```python
from build123d import *

# Parameters (mm, degrees)
SKETCH_1_W             = 6
SKETCH_1_H             = 43
EXTRUDE_1_DEPTH        = 10
SKETCH_3_R             = 1
EXTRUDE_2_DEPTH        = 3
FILLET_1_R             = 1
SKETCH_4_W             = 0.5
SKETCH_4_H             = 2
SKETCH_4_W_2           = 2
SKETCH_4_H_2           = 0.5
CUT_EXTRUDE_1_DEPTH    = 4
SKETCH_5_OUTSIDE_W     = 17.062
SKETCH_5_OUTSIDE_H     = 54.062
CUT_EXTRUDE_2_DEPTH    = 7
CUT_EXTRUDE_3_DEPTH    = 7
SKETCH_7_W             = 3.5
SKETCH_7_H             = 36
CUT_EXTRUDE_4_DEPTH    = 2
CHAMFER_1_SIZE         = 2
CHAMFER_1_SIZE2        = 0.5
CHAMFER_1_PART_2_SIZE  = 2
CHAMFER_1_PART_2_SIZE2 = 0.5
CHAMFER_2_SIZE         = 2
CHAMFER_2_SIZE2        = 0.5
CHAMFER_2_PART_2_SIZE  = 2
CHAMFER_2_PART_2_SIZE2 = 0.5
CHAMFER_3_SIZE         = 2
CHAMFER_3_SIZE2        = 1
CHAMFER_3_PART_2_SIZE  = 2
CHAMFER_3_PART_2_SIZE2 = 1
CHAMFER_4_SIZE         = 0.5
CHAMFER_4_SIZE2        = 1
CHAMFER_4_PART_2_SIZE  = 0.5
CHAMFER_4_PART_2_SIZE2 = 1


with BuildPart() as part:
    # 草图1 → 凸台-拉伸1 (new body)
    with BuildSketch(Plane(origin=(0, 0, 0), x_dir=(1, 0, 0), z_dir=(0, 1, 0))):
        Rectangle(SKETCH_1_W, SKETCH_1_H)
    extrude(amount=EXTRUDE_1_DEPTH)

    # 草图3 → 凸台-拉伸2 (add)
    with BuildSketch(Plane.XZ):
        with Locations((0, 19.5)):
            Circle(SKETCH_3_R)
        with Locations((0, -19.5)):
            Circle(SKETCH_3_R)
    extrude(amount=EXTRUDE_2_DEPTH)

    # 圆角1
    fillet_1_edges = [part.edges().sort_by_distance(p)[0] for p in [
        (-1, -3, 19.5),
        (-1, -3, -19.5),
    ]]
    fillet(fillet_1_edges, radius=FILLET_1_R)

    # 草图4 → 切除-拉伸1 (cut, through all)
    with BuildSketch(Plane.XZ):
        with Locations((0, 19.5)):
            Rectangle(SKETCH_4_W, SKETCH_4_H)
        with Locations((0, -19.5)):
            Rectangle(SKETCH_4_W_2, SKETCH_4_H_2)
    extrude(amount=CUT_EXTRUDE_1_DEPTH, mode=Mode.SUBTRACT)

    # 草图5 outside → 切除-拉伸2 (cut)
    with BuildSketch(Plane(origin=(0, 10, 0), x_dir=(1, 0, 0), z_dir=(0, 1, 0))):
        Rectangle(SKETCH_5_OUTSIDE_W, SKETCH_5_OUTSIDE_H)
        Polygon((-0.75, -20.25), (0.75, -20.25), (0.75, -18), (1.75, -18), (1.75, 18), (0.75, 18), (0.75, 20.25), (-0.75, 20.25), (-0.75, 18), (-1.75, 18), (-1.75, -18), (-0.75, -18), align=None, mode=Mode.SUBTRACT)
    extrude(amount=-CUT_EXTRUDE_2_DEPTH, mode=Mode.SUBTRACT)

    # 草图6 → 切除-拉伸3 (cut)
    with BuildSketch(Plane(origin=(0, 10, 0), x_dir=(1, 0, 0), z_dir=(0, 1, 0))):
        Polygon((-1.25, 17), (0.25, 17), (0.25, -2.5), (1.45, -2.5), (1.45, -4), (-1.25, -4), align=None)
        Polygon((-1.25, -17), (0.25, -17), (0.25, -7.5), (1.45, -7.5), (1.45, -6), (-1.25, -6), align=None)
    extrude(amount=-CUT_EXTRUDE_3_DEPTH, mode=Mode.SUBTRACT)

    # 草图7 → 切除-拉伸4 (cut)
    with BuildSketch(Plane(origin=(0, 10, 0), x_dir=(1, 0, 0), z_dir=(0, 1, 0))):
        Rectangle(SKETCH_7_W, SKETCH_7_H)
    extrude(amount=-CUT_EXTRUDE_4_DEPTH, mode=Mode.SUBTRACT)

    # 倒角1
    chamfer_1_edges = [part.edges().sort_by_distance(p)[0] for p in [
        (0.75, 10, -19.125),
    ]]
    chamfer_1_side = [part.faces().sort_by_distance(p)[0] for p in [
        (0.75, 6.5, -19.125),
    ]]
    chamfer(chamfer_1_edges, length=CHAMFER_1_SIZE, length2=CHAMFER_1_SIZE2, reference=chamfer_1_side[0])

    # 倒角1 part 2
    chamfer_1_part_2_edges = [part.edges().sort_by_distance(p)[0] for p in [
        (-0.75, 10, -19.125),
    ]]
    chamfer_1_part_2_side = [part.faces().sort_by_distance(p)[0] for p in [
        (-0.75, 6.5, -19.125),
    ]]
    chamfer(chamfer_1_part_2_edges, length=CHAMFER_1_PART_2_SIZE, length2=CHAMFER_1_PART_2_SIZE2, reference=chamfer_1_part_2_side[0])

    # 倒角2
    chamfer_2_edges = [part.edges().sort_by_distance(p)[0] for p in [
        (0.75, 10, 19.125),
    ]]
    chamfer_2_side = [part.faces().sort_by_distance(p)[0] for p in [
        (0.75, 6.5, 19.125),
    ]]
    chamfer(chamfer_2_edges, length=CHAMFER_2_SIZE, length2=CHAMFER_2_SIZE2, reference=chamfer_2_side[0])

    # 倒角2 part 2
    chamfer_2_part_2_edges = [part.edges().sort_by_distance(p)[0] for p in [
        (-0.75, 10, 19.125),
    ]]
    chamfer_2_part_2_side = [part.faces().sort_by_distance(p)[0] for p in [
        (-0.75, 6.5, 19.125),
    ]]
    chamfer(chamfer_2_part_2_edges, length=CHAMFER_2_PART_2_SIZE, length2=CHAMFER_2_PART_2_SIZE2, reference=chamfer_2_part_2_side[0])

    # 倒角3
    chamfer_3_edges = [part.edges().sort_by_distance(p)[0] for p in [
        (0, 10, -20.25),
    ]]
    chamfer_3_side = [part.faces().sort_by_distance(p)[0] for p in [
        (0, 6.201754386, -20.25),
    ]]
    chamfer(chamfer_3_edges, length=CHAMFER_3_SIZE, length2=CHAMFER_3_SIZE2, reference=chamfer_3_side[0])

    # 倒角3 part 2
    chamfer_3_part_2_edges = [part.edges().sort_by_distance(p)[0] for p in [
        (0, 10, 20.25),
    ]]
    chamfer_3_part_2_side = [part.faces().sort_by_distance(p)[0] for p in [
        (0, 6.201754386, 20.25),
    ]]
    chamfer(chamfer_3_part_2_edges, length=CHAMFER_3_PART_2_SIZE, length2=CHAMFER_3_PART_2_SIZE2, reference=chamfer_3_part_2_side[0])

    # 倒角4
    chamfer_4_edges = [part.edges().sort_by_distance(p)[0] for p in [
        (0, 10, -18),
    ]]
    chamfer_4_side = [part.faces().sort_by_distance(p)[0] for p in [
        (0, 10, -18.625),
    ]]
    chamfer(chamfer_4_edges, length=CHAMFER_4_SIZE, length2=CHAMFER_4_SIZE2, reference=chamfer_4_side[0])

    # 倒角4 part 2
    chamfer_4_part_2_edges = [part.edges().sort_by_distance(p)[0] for p in [
        (0, 10, 18),
    ]]
    chamfer_4_part_2_side = [part.faces().sort_by_distance(p)[0] for p in [
        (0, 10, 18.625),
    ]]
    chamfer(chamfer_4_part_2_edges, length=CHAMFER_4_PART_2_SIZE, length2=CHAMFER_4_PART_2_SIZE2, reference=chamfer_4_part_2_side[0])


solid = part.part
```
The model under review builds one solid part; all positions refer to its coordinate system, in mm. A direction names the side the tool comes from. Give positions to 0.01 mm unless a question says otherwise; leave off trailing zeros. Write each loop counter-clockwise with the first axis right and the second up, starting at its lowest first coordinate (ties: lowest second). Pieces come first, ordered by that corner, then holes. Notation, with made-up numbers: M -8.5,1.25 L 28.5,1.25 A6 ccw 28.5,5.25 Z; hole C -8,73 d9. An arc over 180 degrees is marked long. Write each question's results on one line, items separated by ' | '. Start each with the question number.
1. Insertion check: pin 1 Ø3 at (x, z) = (0.5, 4) entering from -Y; pin 2 Ø1.4 at (x, y) = (1, 6.5) entering from -Z; pin 3 Ø0.5 at (x, y) = (1.5, 6.5) entering from -Z. Each pin has a flat end and moves straight along its axis. Give the tip position at first contact, or say it passes through.
2. For probe 1 along X at (y, z) = (4.25, 10); probe 2 along Y at (x, z) = (0.6, 3.5); probe 3 along Y at (x, z) = (1.1, -10), list the stretches that pass through material, from the lowest coordinate up. Write a range as [from, to].
3. For faces 1 (the flat face through (-1.25, 6, -6)), 2 (the cylindrical face through (0, -1, -18.5)), 3 (the flat face through (1.75, 6, 0)), 4 (the flat face through (0.25, -1, 19)), 5 (the flat face through (0, 9.4, -18.2)), list the 3-axis set-ups (+Z, -Z, +X, -X, +Y, -Y) from which the entire face can be reached by the end or side of a thin tool; tool diameter is ignored.
4. Mouldability with a two-part tool opening along Z and no side actions: class faces 6 (the flat face through (0.552, 8.792, 18.891)), 7 (the flat face through (0, -1, -19.25)), 8 (the flat face through (1, 6, -18)) as released by +Z, released by -Z, zero draft, split by the parting line, or undercut.
5. We need section B-B (z = 8). Write out the cut boundary in (x, y), and give its area (3 significant figures).
6. We need section C-C (x = -2.5). Write out the cut boundary in (y, z).
7. We need section A-A (y = 7). Write out the cut boundary in (x, z), and give its area (4 significant figures).
Results found:
1) pin 1: stops at y = 0 | pin 2: stops at z = -20.25 | pin 3: stops at z = -18
2) probe 1: x = [-1.75, -1.25], [0.25, 1.75] | probe 2: y = [0, 3] | probe 3: y = [0, 8]
3) face 1: +Y | face 2: -Y | face 3: +Z, -Z, +X, +Y | face 4: +Z, -Y | face 5: +X, -X, +Y
4) face 6: zero draft | face 7: undercut | face 8: released by -Z
5) outline: M -3,0 L 3,0 L 3,3 L 1.75,3 L 1.75,8 L 0.25,8 L 0.25,3 L -1.25,3 L -1.25,8 L -1.75,8 L -1.75,3 L -3,3 Z | area: 28.0 mm^2
6) outline: M 0,-21.5 L 3,-21.5 L 3,21.5 L 0,21.5 Z
7) outline: M -1.75,-18 L -0.75,-18 L -0.75,-20.25 L 0.75,-20.25 L 0.75,-18 L 1.75,-18 L 1.75,18 L 0.75,18 L 0.75,20.25 L -0.75,20.25 L -0.75,18 L -1.75,18 Z; hole M -1.25,-17 L 0.25,-17 L 0.25,2.5 L 1.45,2.5 L 1.45,4 L -1.25,4 Z; hole M -1.25,6 L 1.45,6 L 1.45,7.5 L 0.25,7.5 L 0.25,17 L -1.25,17 Z | area: 81.15 mm^2
